Part model, mm, in its own coordinate system. Face numbers are marked on the shaded views. A direction names the side the tool comes from. Round coordinates to 2 decimals unless told otherwise and drop trailing zeros. Loops run counter-clockwise (first coordinate to the right, second up) from the corner with the lowest first, then second, coordinate; pieces in that order, holes last.
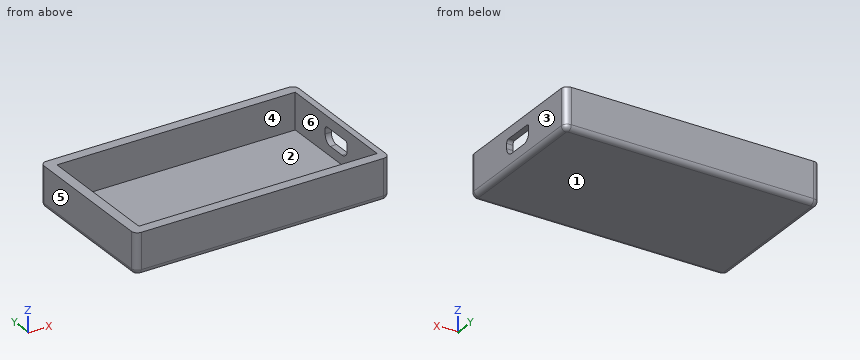
from build123d import *

# Parameters (mm, degrees)
F0_W     = 62.5
F0_H     = 36.5
F0_W_2   = 58.5
F0_H_2   = 31.5
F1_DEPTH = 10
F2_DEPTH = 1.1
F3_R     = 1.5
F4_R     = 1.2
F6_DEPTH = 3


with BuildPart() as f1:
    # F0 (on Top) → F1 (new body)
    with BuildSketch(Plane.XY):
        with Locations((0.005647, 0.384062)):
            Rectangle(F0_W, F0_H)
        with Locations((0.505647, 0.384062)):
            Rectangle(F0_W_2, F0_H_2, mode=Mode.SUBTRACT)
    extrude(amount=F1_DEPTH)

    # F0 (on Top) → F2 (join)
    with BuildSketch(Plane.XY):
        with Locations((0.505647, 0.384062)):
            Rectangle(F0_W_2, F0_H_2)
    extrude(amount=F2_DEPTH)

    # F3
    f3_edges = [f1.edges().sort_by_distance(p)[0] for p in [
        (31.255647, -17.865938, 5),
        (31.255647, 18.634062, 5),
        (-31.244353, 18.634062, 5),
        (-31.244353, -17.865938, 5),
    ]]
    fillet(f3_edges, radius=F3_R)

    # F4
    f4_edges = [f1.edges().sort_by_distance(p)[0] for p in [
        (0.005647, 18.634062, 0),
        (30.816307, 18.194723, 0),
        (-30.805013, 18.194723, 0),
        (31.255647, 0.384062, 0),
        (-31.244353, 0.384062, 0),
        (30.816307, -17.426598, 0),
        (-30.805013, -17.426598, 0),
        (0.005647, -17.865938, 0),
    ]]
    fillet(f4_edges, radius=F4_R)

    # F5 (on face) → F6 (cut)
    with BuildSketch(Plane.YZ.offset(31.255647)):
        with BuildLine():
            Line((3.884062, 7.420129), (-3.115938, 7.420129))
            ThreePointArc((-3.115938, 7.420129), (-3.646268, 7.200459), (-3.865938, 6.670129))
            Line((-3.865938, 6.670129), (-3.865938, 5.420129))
            ThreePointArc((-3.865938, 5.420129), (-3.280151, 4.005916), (-1.865938, 3.420129))
            Line((-1.865938, 3.420129), (2.634062, 3.420129))
            ThreePointArc((2.634062, 3.420129), (4.048276, 4.005916), (4.634062, 5.420129))
            Line((4.634062, 5.420129), (4.634062, 6.670129))
            ThreePointArc((4.634062, 6.670129), (4.414393, 7.200459), (3.884062, 7.420129))
        make_face()
    extrude(amount=-F6_DEPTH, mode=Mode.SUBTRACT)


solid = f1.part
1) Mould opens along X. For the marked faces 1, 2, 3 and 4 say: released by +X, released by -X, zero draft, split by the parting line, or undercut.
Values:
face 1: zero draft
face 2: undercut
face 3: released by +X
face 4: undercut
2) Drop a flat-ended pin along its axis: pin 1 Ø4 at (x, y) = (9, -1.5) entering from +Z. Give the stop position or say it passes through.
Values:
pin 1: stops at z = 1.1
3) Wall check: line 1 along X through (y, z) = (-0.5, 2.25); line 2 along Y through (x, z) = (-4.5, 1.5); line 3 along Z through (x, y) = (10, 7). Give the ranges that are in metal, low to high.
Values:
line 1: x = -31.24 to -28.74, 29.76 to 31.26
line 2: y = -17.87 to -15.37, 16.13 to 18.63
line 3: z = 0 to 1.1
4) Slice it at D-D, the plane y = 11.5. Give the cut face in (x, z), then the cut area to 3 significant figures.
Values:
outline: (-31.24, 1.2) arc R1.2 ccw to (-30.04, 0) - (30.06, 0) arc R1.2 ccw to (31.26, 1.2) - (31.26, 10) - (29.76, 10) - (29.76, 1.1) - (-28.74, 1.1) - (-28.74, 10) - (-31.24, 10) - close
area: 104 mm2
5) Slice it at A-A, the plane y = 1.5. Give the cut face in (x, z), then the cut area to 3 significant figures.
Values:
outline: (-31.24, 1.2) arc R1.2 ccw to (-30.04, 0) - (30.06, 0) arc R1.2 ccw to (31.26, 1.2) - (31.26, 3.42) - (29.76, 3.42) - (29.76, 1.1) - (-28.74, 1.1) - (-28.74, 10) - (-31.24, 10) - close; (29.76, 7.42) - (31.26, 7.42) - (31.26, 10) - (29.76, 10) - close
area: 97.7 mm2
6) Slice it at C-C, the plane z = 8.5. Give the cut face in (x, y).
Values:
outline: (-31.24, -16.37) arc R1.5 ccw to (-29.74, -17.87) - (29.76, -17.87) arc R1.5 ccw to (31.26, -16.37) - (31.26, 17.13) arc R1.5 ccw to (29.76, 18.63) - (-29.74, 18.63) arc R1.5 ccw to (-31.24, 17.13) - close; hole (-28.74, -15.37) - (29.76, -15.37) - (29.76, 16.13) - (-28.74, 16.13) - close
7) Slice it at B-B, the plane x = 11. Give the cut face in (y, z), then the cut area to 3 significant figures.
Values:
outline: (-17.87, 1.2) arc R1.2 ccw to (-16.67, 0) - (17.43, 0) arc R1.2 ccw to (18.63, 1.2) - (18.63, 10) - (16.13, 10) - (16.13, 1.1) - (-15.37, 1.1) - (-15.37, 10) - (-17.87, 10) - close
area: 84.0 mm2
8) Tool access for the marked faces 5 and 6: list every direction of +Z, -Z, +X, -X, +Y, -Y with a clear straight run to the whole face (end or side of a thin tool).
Values:
face 5: +Z, -Z, -X, +Y, -Y
face 6: +Z
